Study the drawing (mm; zero at the part's minimum x, y, z) and answer. A direction names the side the tool comes from. Coordinates: 2 decimals unless noted, no trailing zeros. Loops run counter-clockwise (first coordinate to the right, second up) from the corner with the lowest first, then second, coordinate; pieces in that order, holes last. Notation, with made-up numbers: (-31, -34.5) - (-19, -34.5) arc R24 cw to (-19, -6.5) - close; hole circle Ø7 at (-13.5, 58). An arc over 180 degrees is marked (long way). Write each question's results on one line, items separated by ' | '. Start each with the question number.
(1) Consider line 1 (X direction, y = 115.5, z = 16); line 2 (Z direction, x = 41, y = 114.5); line 3 (Z direction, x = 113, y = 14) (3 decimals). Determine where each line is inside the solid, lowest interval first. Write a range as from..to.
(2) Determine the mould class of the marked faces 1, 2, 3 and 4 for opening direction X: released by +X, released by -X, zero draft, split by the parting line, or undercut.
(3) For the marked faces 5, 6 and 7, determine the directions among +Z, -Z, +X, -X, +Y, -Y from which every point of the face is accessible in a straight line to the end or side of a thin tool.
(4) Given pin 1 Ø18.5 at (y, z) = (83.5, 10) entering from +X; pin 2 Ø5.5 at (y, z) = (73, 50.5) entering from -X; pin 3 Ø5 at (x, y) = (49.5, 28.5) entering from -Z; pin 4 Ø2.5 at (y, z) = (73, 74.5) entering from -X, each flat-ended and moving along its own axis, determine where each tip first touches the part or whether it passes through.
(5) Find section C-C on z = 43. Determine the outline of the cut face in (x, y).
(6) Find section B-B on x = 49. Determine the outline of the cut face in (y, z).
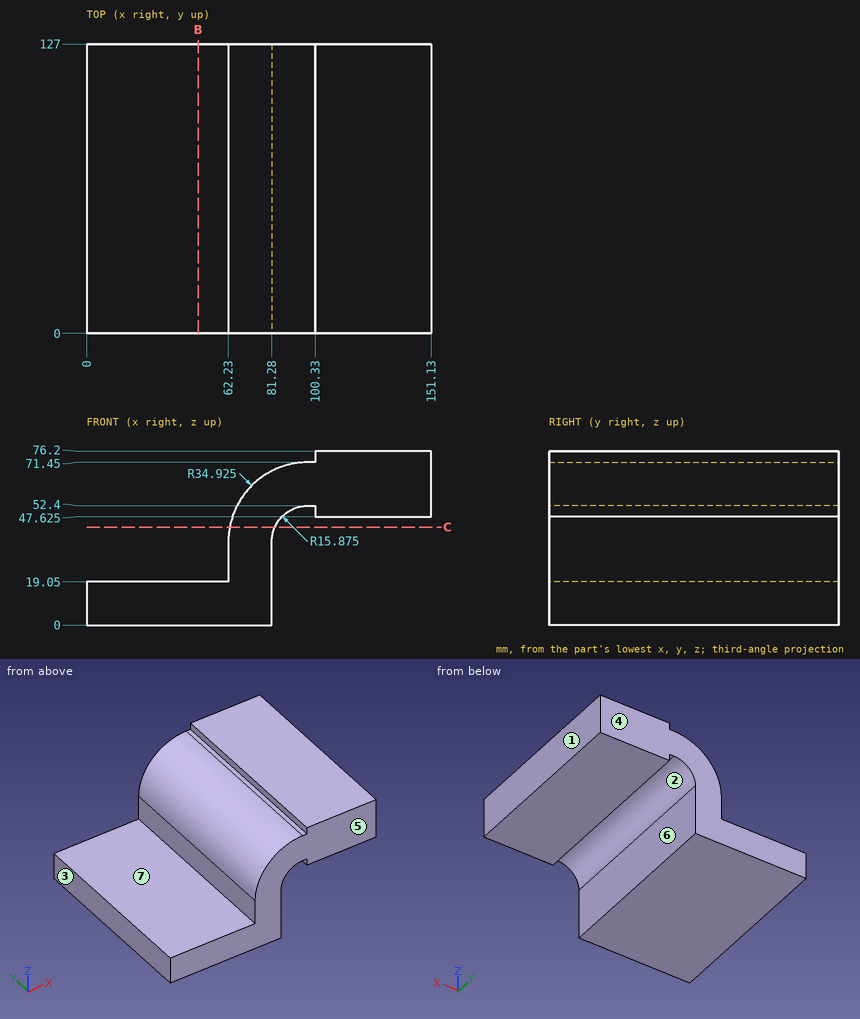
Values:
1) line 1: x = 0..81.28 | line 2: z = 0..19.05 | line 3: z = 47.625..76.2
2) face 1: released by +X | face 2: undercut | face 3: released by -X | face 4: zero draft
3) face 5: +Z, -Z, +X, -X, -Y | face 6: -Z, +X, +Y, -Y | face 7: +Z, -X, +Y, -Y
4) pin 1: stops at x = 81.28 | pin 2: stops at x = 64.08 | pin 3: stops at z = 0 | pin 4: stops at x = 100.33
5) outline: (62.84, 0) - (82.66, 0) - (82.66, 127) - (62.84, 127) - close
6) outline: (0, 0) - (127, 0) - (127, 19.05) - (0, 19.05) - close
